Drawing for the job (mm, zero at the part's lowest x, y, z). A direction names the side the tool comes from. Round coordinates to 2 decimals unless told otherwise and drop trailing zeros. Loops run counter-clockwise (first coordinate to the right, second up) from the corner with the lowest first, then second, coordinate; pieces in that order, holes last. Notation, with made-up numbers: M -0.75,84 L 39.25,84 A22 ccw 39.25,111 Z; hole C 86,22.5 d7. An arc over 180 degrees is marked long. Answer in a Markdown table with one row per item.
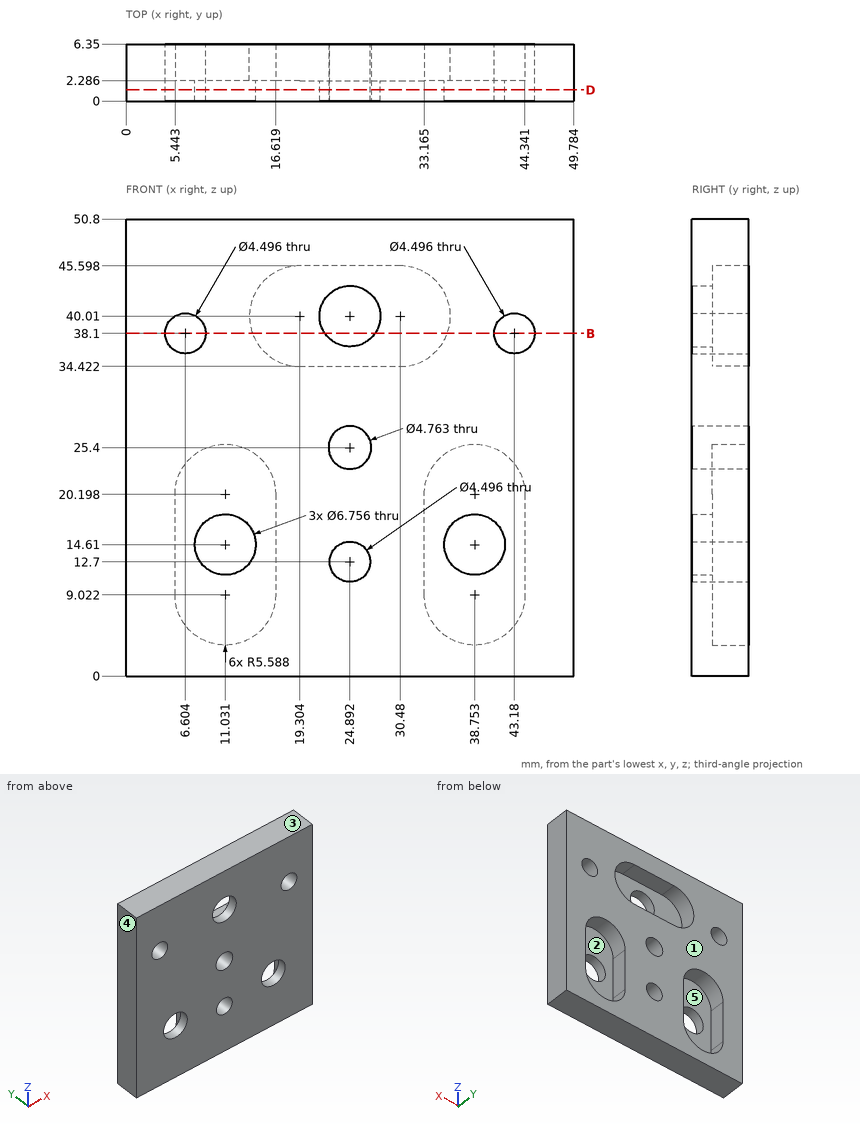
1. Saw through at D-D (y = 1.25). Write the cut outline in (x, z) (1 decimal), and give its area (3 significant figures).
Verdict:
| item | result |
|---|---|
| outline | M 0,0 L 49.8,0 L 49.8,50.8 L 0,50.8 Z; hole C 6.6,38.1 d4.5; hole C 11,14.6 d6.8; hole C 24.9,40 d6.8; hole C 24.9,25.4 d4.8; hole C 24.9,12.7 d4.5; hole C 38.8,14.6 d6.8; hole C 43.2,38.1 d4.5 |
| area | 2,360 mm² |
2. Pin check, flat tip, straight feed: pin 1 (11 mm diameter, centred on x = 38.75, z = 14.61, fed in from +Y). Stop position of the tip, or through.
Verdict:
| item | result |
|---|---|
| pin 1 | stops at y = 2.29 |
3. Mould opens along X. For the marked faces 3, 4 and 5 say: +X half, -X half, draft (parallel to the pull), parting line (faces both ways), or undercut.
Verdict:
| item | result |
|---|---|
| face 3 | draft |
| face 4 | -X half |
| face 5 | undercut |
4. Wall check: probe 1 along X at (y, z) = (5, 9) (1 decimal); probe 2 along X at (y, z) = (1.75, 25.4) (1 decimal); probe 3 along Z at (x, y) = (25, 5.5) (1 decimal). Give the ranges that are in metal, low to high.
Verdict:
| item | result |
|---|---|
| probe 1 | x = 0 to 5.4, 16.6 to 33.2, 44.3 to 49.8 |
| probe 2 | x = 0 to 22.5, 27.3 to 49.8 |
| probe 3 | z = 0 to 10.5, 14.9 to 23, 27.8 to 34.4, 45.6 to 50.8 |
5. Tool access for the marked faces 1 and 2: list every direction of +Z, -Z, +X, -X, +Y, -Y with a clear straight run to the whole face (end or side of a thin tool).
Verdict:
| item | result |
|---|---|
| face 1 | +Z, -Z, +X, -X, +Y |
| face 2 | +Y |
6. Saw through at B-B (z = 38.1). State how many separate pieces and enclosed holes the cut face has, and give its area (3 significant figures).
Verdict:
| item | result |
|---|---|
| separate pieces | 4 |
| enclosed holes | 0 |
| area | 158 mm² |
